from build123d import *

# Parameters (mm, degrees)
SKETCH1_W           = 127
SKETCH1_H           = 127
BOSS_EXTRUDE1_DEPTH = 5.08
CUT_EXTRUDE1_REACH  = 91.946
SKETCH2_R           = 5.3467
SKETCH4_R           = 9.017
SKETCH4_R_2         = 7.62
CUT_EXTRUDE3_DEPTH  = 0.9779
SKETCH5_R           = 1.03251
CUT_EXTRUDE4_DEPTH  = 3.175
CIRPATTERN1_COUNT   = 6
CUT_EXTRUDE5_REACH  = 91.946
SKETCH6_R           = 1.63195
CIRPATTERN2_COUNT   = 9
CUT_EXTRUDE6_REACH  = 91.946
SKETCH7_R           = 3.175
SKETCH9_R           = 10.9855
SKETCH9_R_2         = 5.3467
BOSS_EXTRUDE2_DEPTH = 1.27


with BuildPart() as part:
    # Sketch1 → Boss-Extrude1 (new body)
    with BuildSketch(Plane(origin=(0, 0, 0), x_dir=(1, 0, 0), z_dir=(0, 1, 0))):
        Rectangle(SKETCH1_W, SKETCH1_H)
    extrude(amount=BOSS_EXTRUDE1_DEPTH)

    # Sketch2 → Cut-Extrude1 (cut, up to next)
    with BuildSketch(Plane(origin=(0, 5.08, 0), x_dir=(1, 0, 0), z_dir=(0, 1, 0)), mode=Mode.PRIVATE) as cut_extrude1_sk1:
        with Locations(Location((0, 0, 0), (0, 0, 270))):
            Circle(SKETCH2_R)
    cut_extrude1_tool1 = extrude(cut_extrude1_sk1.sketch, amount=-CUT_EXTRUDE1_REACH, mode=Mode.PRIVATE) & part.part
    add(cut_extrude1_tool1.solids().sort_by_distance((0, 5.08, 0))[0], mode=Mode.SUBTRACT)

    # Sketch4 → Cut-Extrude3 (cut)
    with BuildSketch(Plane(origin=(0, 5.08, 0), x_dir=(1, 0, 0), z_dir=(0, 1, 0))):
        with Locations(Location((0, 0, 0), (0, 0, 270))):
            Circle(SKETCH4_R)
        with Locations(Location((0, 0, 0), (0, 0, 270))):
            Circle(SKETCH4_R_2, mode=Mode.SUBTRACT)
    extrude(amount=-CUT_EXTRUDE3_DEPTH, mode=Mode.SUBTRACT)

    # Sketch5 → Cut-Extrude4 (cut)
    with BuildSketch(Plane(origin=(0, 5.08, 0), x_dir=(1, 0, 0), z_dir=(0, 1, 0))):
        with Locations(Location((0, -15.24, 0), (0, 0, 270))):
            Circle(SKETCH5_R)
    cut_extrude4 = extrude(amount=-CUT_EXTRUDE4_DEPTH, mode=Mode.SUBTRACT)

    # CirPattern1: Cut-Extrude4 ×6 about axis
    cirpattern1_axis = Axis((0, 0, 0), (0, 1, 0))
    for i in range(1, CIRPATTERN1_COUNT):
        add(cut_extrude4.rotate(cirpattern1_axis, i * 360 / CIRPATTERN1_COUNT), mode=Mode.SUBTRACT)

    # Sketch6 → Cut-Extrude5 (cut, up to next)
    with BuildSketch(Plane(origin=(0, 5.08, 0), x_dir=(1, 0, 0), z_dir=(0, 1, 0)), mode=Mode.PRIVATE) as cut_extrude5_sk1:
        with Locations(Location((22.225, -38.494829198, 0), (0, 0, 270))):
            Circle(SKETCH6_R)
    cut_extrude5_tool1 = extrude(cut_extrude5_sk1.sketch, amount=-CUT_EXTRUDE5_REACH, mode=Mode.PRIVATE) & part.part
    cut_extrude5 = cut_extrude5_tool1.solids().sort_by_distance((22.225, 5.08, 38.494829))[0]
    add(cut_extrude5, mode=Mode.SUBTRACT)

    # CirPattern2: Cut-Extrude5 ×9 about axis
    cirpattern2_axis = Axis((0, 0, 0), (0, 1, 0))
    for i in range(1, CIRPATTERN2_COUNT):
        add(cut_extrude5.rotate(cirpattern2_axis, i * 360 / CIRPATTERN2_COUNT), mode=Mode.SUBTRACT)

    # Sketch7 → Cut-Extrude6 (cut, up to next)
    with BuildSketch(Plane(origin=(0, 5.08, 0), x_dir=(1, 0, 0), z_dir=(0, 1, 0)), mode=Mode.PRIVATE) as cut_extrude6_sk1:
        with Locations(Location((57.15, 57.15, 0), (0, 0, 270))):
            Circle(SKETCH7_R)
    cut_extrude6_tool1 = extrude(cut_extrude6_sk1.sketch, amount=-CUT_EXTRUDE6_REACH, mode=Mode.PRIVATE) & part.part
    # Sketch7 → Cut-Extrude6 (cut, up to next)
    with BuildSketch(Plane(origin=(0, 5.08, 0), x_dir=(1, 0, 0), z_dir=(0, 1, 0)), mode=Mode.PRIVATE) as cut_extrude6_sk2:
        with Locations(Location((57.15, -57.15, 0), (0, 0, 90))):
            Circle(SKETCH7_R)
    cut_extrude6_tool2 = extrude(cut_extrude6_sk2.sketch, amount=-CUT_EXTRUDE6_REACH, mode=Mode.PRIVATE) & part.part
    # Sketch7 → Cut-Extrude6 (cut, up to next)
    with BuildSketch(Plane(origin=(0, 5.08, 0), x_dir=(1, 0, 0), z_dir=(0, 1, 0)), mode=Mode.PRIVATE) as cut_extrude6_sk3:
        with Locations(Location((-57.15, -57.15, 0), (0, 0, 270))):
            Circle(SKETCH7_R)
    cut_extrude6_tool3 = extrude(cut_extrude6_sk3.sketch, amount=-CUT_EXTRUDE6_REACH, mode=Mode.PRIVATE) & part.part
    # Sketch7 → Cut-Extrude6 (cut, up to next)
    with BuildSketch(Plane(origin=(0, 5.08, 0), x_dir=(1, 0, 0), z_dir=(0, 1, 0)), mode=Mode.PRIVATE) as cut_extrude6_sk4:
        with Locations(Location((-57.15, 57.15, 0), (0, 0, 90))):
            Circle(SKETCH7_R)
    cut_extrude6_tool4 = extrude(cut_extrude6_sk4.sketch, amount=-CUT_EXTRUDE6_REACH, mode=Mode.PRIVATE) & part.part
    add(cut_extrude6_tool1.solids().sort_by_distance((57.15, 5.08, -57.15))[0], mode=Mode.SUBTRACT)
    add(cut_extrude6_tool2.solids().sort_by_distance((57.15, 5.08, 57.15))[0], mode=Mode.SUBTRACT)
    add(cut_extrude6_tool3.solids().sort_by_distance((-57.15, 5.08, 57.15))[0], mode=Mode.SUBTRACT)
    add(cut_extrude6_tool4.solids().sort_by_distance((-57.15, 5.08, -57.15))[0], mode=Mode.SUBTRACT)

    # Sketch9 → Boss-Extrude2 (add)
    with BuildSketch(Plane.XZ):
        with Locations(Location((0, 0, 0), (0, 0, 270))):
            Circle(SKETCH9_R)
        with Locations(Location((0, 0, 0), (0, 0, 90))):
            Circle(SKETCH9_R_2, mode=Mode.SUBTRACT)
    extrude(amount=BOSS_EXTRUDE2_DEPTH)


solid = part.part
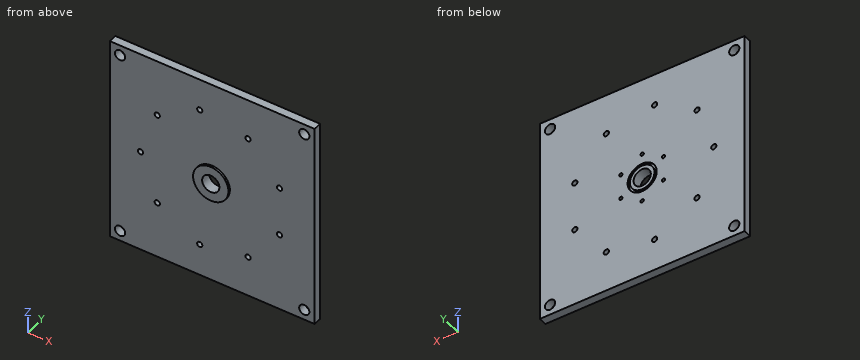
Read the model definition and answer for the solid it produces. Units are mm, in the model's axes. Give positions to 0.01 mm unless a question says otherwise; leave off trailing zeros. Write each loop counter-clockwise with the first axis right and the second up, starting at its lowest first coordinate (ties: lowest second). Pieces come first, ordered by that corner, then holes. Notation, with made-up numbers: (67.5, 68) - (104.5, 68) arc R25 cw to (104.5, 105) - close; hole circle Ø2 at (28, 87). An arc over 180 degrees is marked (long way). Use CSV: the item, a comma, the result in double quotes. Start each with the question number.
Item 1: The part is cut by section C-C, the plane y = 3. Count the separate pieces of the cut face and the enclosed holes in it, and give its area (3 significant figures).
Item 2: The part is cut by section D-D, the plane x = -23.5. Give the vertices of the cut face in (y, z).
Item 3: The part is cut by section B-B, the plane z = 57.15. Give the vertices of the cut face in (x, y) (3 decimals).
Item 4: Consider line 1 (X direction, y = 1.6, z = 57.15) (3 decimals); line 2 (X direction, y = 3.4, z = -7.62); line 3 (Z direction, x = -0.5, y = 1.5). Determine where each line is inside the solid, lowest interval first.
Item 5: The part is cut by section A-A, the plane x = -57.15. Give the vertices of the cut face in (y, z) (3 decimals), and give its area (3 significant figures).
Item 6: Flat-ended cylindrical pins translate along their axes: P1, Ø4, axis at x = 22.22, z = 38.49, coming from the -Y side; P2, Ø5.5, axis at x = 57.15, z = 57.15, coming from the -Y side; P3, Ø14, axis at x = 0, z = 0, coming from the -Y side; P4, Ø0.6, axis at x = -0.5, z = 15.5, coming from the +Y side (3 decimals). Find the tip coordinate at first contact, or state that the pin passes through.
Taken from the geometry:
1,separate pieces,"1"
1,enclosed holes,"20"
1,area,"15,800 mm2"
2,outline,"(0, -63.5) - (5.08, -63.5) - (5.08, 63.5) - (0, 63.5) - close"
3,outline,"(-63.5, 0) - (-60.325, 0) - (-60.325, 5.08) - (-63.5, 5.08) - close; (-53.975, 0) - (53.975, 0) - (53.975, 5.08) - (-53.975, 5.08) - close; (60.325, 0) - (63.5, 0) - (63.5, 5.08) - (60.325, 5.08) - close"
4,line 1,"-63.5 to -60.325, -53.975 to 53.975, 60.325 to 63.5"
4,line 2,"-63.5 to -14.23, -12.17 to 12.17, 14.23 to 63.5"
4,line 3,"-63.5 to -5.32, 5.32 to 63.5"
5,outline,"(0, -63.5) - (5.08, -63.5) - (5.08, -60.325) - (0, -60.325) - close; (0, -53.975) - (5.08, -53.975) - (5.08, 53.975) - (0, 53.975) - close; (0, 60.325) - (5.08, 60.325) - (5.08, 63.5) - (0, 63.5) - close"
5,area,"581 mm2"
6,P1,"y = 0"
6,P2,"through"
6,P3,"y = -1.27"
6,P4,"y = 1.905"
